```python
from build123d import *
from build123d import SkipClean  # not in build123d's __all__

# Parameters (mm, degrees)
F0_R        = 7.25
F0_R_2      = 2.5
F1_DEPTH    = 40
F4_S5_R     = 10.75
F4_T6_DEPTH = 17


# Not quite as in the source:
# - a fillet or chamfer that OpenCascade refuses, or shapes differently, is made with other operations: its cross-section is extruded or revolved along the edge and cut away or added


with BuildPart() as f1:
    # F0 (on Top) → F1 (new body)
    with BuildSketch(Plane.XY):
        Circle(F0_R)
        Circle(F0_R_2, mode=Mode.SUBTRACT)
    extrude(amount=F1_DEPTH)

    # F2 (on Front) → F3 (revolve)
    with BuildSketch(Plane.XZ):
        with BuildLine():
            Line((10.75, 3), (2.5, 3))
            Line((2.5, 3), (2.5, 0))
            Line((2.5, 0), (9.75, 0))
            ThreePointArc((9.75, 0), (10.0428932188, 0.7071067812), (10.75, 1))
            Line((10.75, 1), (10.75, 3))
        make_face()
    revolve(axis=Axis((0, 0, 1.5), (0, 0, 1)))

    # F4: chamfer of 4 x 1 on 1 edges, made by hand


with BuildPart() as f4_tool2:
    # F4_s3 → F4_t4 (revolve)
    with BuildSketch(Plane.XZ):
        Polygon((11.25, 3), (7.25, 4), (7.25, 3), align=None)
    revolve(axis=Axis((0, 0, 3), (0, 0, -1)))

    # F4_s5 → F4_t6 (intersect, symmetric)
    with BuildSketch(Plane.XY.offset(3.5)):
        Circle(F4_S5_R)
    extrude(amount=F4_T6_DEPTH, both=True, mode=Mode.INTERSECT)


with BuildPart() as f1_1:
    add(f1.part, clean=False)

    # F4_t1: union F4_tool2
    add(f4_tool2.part)

    # F5: F1 across face


with BuildPart() as f1_2:
    add(f1_1.part, clean=False)
    with SkipClean():  # cleaning this boolean's faces spoils the solid; the shape is the same uncleaned
        add(f1_1.part.mirror(Plane(origin=(0, 0, 0), x_dir=(1, 0, 0), z_dir=(0, 0, -1))), clean=False)


solid = f1_2.part
```
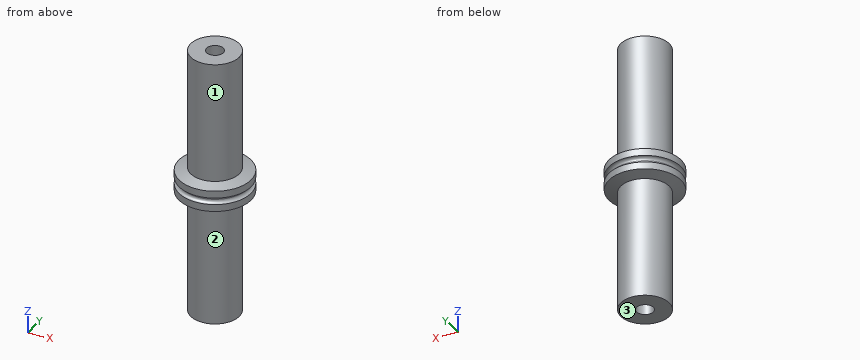
The listing builds one solid part. Answer for the finished solid, in the listing's coordinates (mm). Face numbers are marked on the shaded views. A direction names the side the tool comes from. Give positions to 0.01 mm unless a question says otherwise; leave off trailing zeros. Order: outer loops, then holes, each group sorted by start corner. A loop starts at its lowest first (then second) coordinate and runs counter-clockwise, first axis right, second up.
Item 1: Find the intervals of material crossed by probe 1 along Y at (x, z) = (0, -2); probe 2 along Y at (x, z) = (0, 5); probe 3 along X at (y, z) = (3.75, 23), in increasing order.
From the geometry:
probe 1: y = -10.75 to -2.5, 2.5 to 10.75
probe 2: y = -7.25 to -2.5, 2.5 to 7.25
probe 3: x = -6.2 to 6.2
Item 2: Which of the six approach directions +Z, -Z, +X, -X, +Y, -Y give full straight-line access (tool end or side, diameter ignored) to the marked faces 1, 2 and 3?
From the geometry:
face 1: +Z
face 2: -Z
face 3: -Z, +X, -X, +Y, -Y
Item 3: Given pin 1 Ø1 at (y, z) = (-2.5, 26.5) entering from -X; pin 2 Ø4 at (x, z) = (-0.5, -12.5) entering from -Y; pin 3 Ø4 at (x, z) = (-5.5, 27.5) entering from -Y, each flat-ended and moving along its own axis, determine where each tip first touches the part or whether it passes through.
From the geometry:
pin 1: stops at x = -6.97
pin 2: stops at y = -7.25
pin 3: stops at y = -6.35
Item 4: The part is cut by section A-A, the plane z = 21. Give the vertices of the cut face in (x, y).
From the geometry:
outline: circle Ø14.5 at (0, 0); hole circle Ø5 at (0, 0)
